Autodesk Inventor part; units mm, degrees
ref_plane "YZ Plane" through (0, 0, 0) normal (1, 0, 0) x (0, 1, 0)
ref_plane "XZ Plane" through (0, 0, 0) normal (0, 1, 0) x (-1, 0, 0)
ref_plane "XY Plane" through (0, 0, 0) normal (0, 0, 1) x (1, 0, 0)
sketch "Sketch1" plane through (0, 0, 0) normal (0, 1, 0) x (-1, 0, 0)
  line L0 (-12.7, -12.7) -> (12.7, -12.7)
  line L1 (12.7, -12.7) -> (12.7, 12.7)
  line L2 (12.7, 12.7) -> (-12.7, 12.7)
  line L3 (-12.7, 12.7) -> (-12.7, -12.7)
  line L4 (-12.7, -12.7) -> (12.7, 12.7) construction
  line L5 (12.7, -12.7) -> (-12.7, 12.7) construction
  line L6 (-10.9728, -10.9728) -> (10.9728, -10.9728)
  line L7 (10.9728, -10.9728) -> (10.9728, 10.9728)
  line L8 (10.9728, 10.9728) -> (-10.9728, 10.9728)
  line L9 (-10.9728, 10.9728) -> (-10.9728, -10.9728)
  line L10 (-10.9728, -10.9728) -> (10.9728, 10.9728) construction
  line L11 (10.9728, -10.9728) -> (-10.9728, 10.9728) construction
  point P0 (0, 0)
  dimension "d0" = 25.4
  dimension "d2" = 25.4
  dimension "d3" = 1.7272
  dimension "d4" = 1.7272
extrude "Extrusion1" add sketch "Sketch1" along normal blind 352.425
sketch "Sketch2" plane through (12.7, 0, 12.7) normal (1, 0, 0) x (0, 0, -1)
  line L0 (0, 352.425) -> (25.4, 352.425)
  line L1 (0, 0) -> (0, 352.425)
  point P0 (12.7, 0)
  point P1 (12.7, 339.725)
  dimension "d7" = 12.7
  dimension "d8" = 12.7
hole "Hole1" at (12.7, 339.725, 0) direction (-1, 0, 0) diameter 6.35 end through all
sketch "Sketch4" plane through (-12.7, 0, 12.7) normal (0, 0, 1) x (1, 0, 0)
  line L0 (0, 0) -> (25.4, 0)
  line L1 (25.4, 0) -> (25.4, 352.425)
  point P0 (12.7, 0)
  point P1 (12.7, 12.7)
  dimension "d25" = 12.7
  dimension "d26" = 12.7
hole "Hole3" at (0, 12.7, 12.7) direction (0, 0, -1) diameter 6.35 end through all
sketch "Sketch5" plane through (12.7, 0, -12.7) normal (0, 0, -1) x (-1, 0, 0)
  line L0 (0, 0) -> (25.4, 0)
  line L1 (25.4, 0) -> (25.4, 352.425)
  line L2 (0, 352.425) -> (25.4, 352.425)
  point P0 (12.7, 0)
  point P1 (12.7, 203.2)
  point P2 (12.7, 152.4)
  dimension "d34" = 50.8
  dimension "d36" = 152.4
  dimension "d38" = 149.225
  dimension "d39" = 352.425
  dimension "d40" = 12.7
  dimension "d41" = 12.7
hole "Hole4" at (0, 203.2, -12.7) at (0, 152.4, -12.7) direction (0, 0, 1) diameter 6.35 end through all
properties part number "BAseBAr" material "Aluminum 6061"
Geometry: final body of the model. Coordinates: model frame, mm. A direction names the side the tool comes from. Give positions to 0.01 mm unless a question says otherwise; leave off trailing zeros. Write each loop counter-clockwise with the first axis right and the second up, starting at its lowest first coordinate (ties: lowest second). Pieces come first, ordered by that corner, then holes. Notation, with made-up numbers: (44, -10.75) -> (61, -10.75) arc R10 cw to (61, 4.25) -> close; hole circle Ø11 at (-31, 26.5). An arc over 180 degrees is marked (long way). Answer as a JSON object with one key per item and string values.
1. Cut plane C-C on y = 12.7. Output: boundary loops of the cut face in (x, z) (3 decimals), and give its area (3 significant figures).
Ans:
{"outline": "(-12.7, -12.7) -> (-3.175, -12.7) -> (-3.175, -10.973) -> (-10.973, -10.973) -> (-10.973, 10.973) -> (-3.175, 10.973) -> (-3.175, 12.7) -> (-12.7, 12.7) -> close; (3.175, -12.7) -> (12.7, -12.7) -> (12.7, 12.7) -> (3.175, 12.7) -> (3.175, 10.973) -> (10.973, 10.973) -> (10.973, -10.973) -> (3.175, -10.973) -> close", "area": "142 mm^2"}
2. Ray query, probe 1 along Y at (x, z) = (0, 11.95) (3 decimals); probe 2 along X at (y, z) = (209, -3.25). Return the intervals inside material, ascending. Write a range as from..to.
Ans:
{"probe 1": "y = 0..9.525, 15.875..149.225, 155.575..200.025, 206.375..352.425", "probe 2": "x = -12.7..-10.97, 10.97..12.7"}
3. Contact query for a flat-ended pin moving along its axis: pin 1 (8.5 mm diameter, centred on y = 339.725, z = 0, fed in from -X). Output: stop coordinate, or through.
Ans:
{"pin 1": "stops at x = -12.7"}
4. Mould query, pull axis Z, two halves, no side actions, for faces 1 (the flat face through (0, 174, -10.973)), 2 (the cylindrical face through (1.22, 206.13, 11.85)), 3 (the flat face through (0, 174, 12.7)). Classes: pulls with the +Z half, pulls with the -Z half, needs draft (parallel to the pull), parting line crosses it, or undercut.
Ans:
{"face 1": "undercut", "face 2": "needs draft", "face 3": "pulls with the +Z half"}
5. Cut plane B-B on z = 6.75. Output: boundary loops of the cut face in (x, y) (3 decimals).
Ans:
{"outline": "(-12.7, 0) -> (-10.973, 0) -> (-10.973, 352.425) -> (-12.7, 352.425) -> close; (10.973, 0) -> (12.7, 0) -> (12.7, 352.425) -> (10.973, 352.425) -> close"}
6. Cut plane A-A on x = -7.5. Output: boundary loops of the cut face in (y, z) (3 decimals).
Ans:
{"outline": "(0, -12.7) -> (352.425, -12.7) -> (352.425, -10.973) -> (0, -10.973) -> close; (0, 10.973) -> (352.425, 10.973) -> (352.425, 12.7) -> (0, 12.7) -> close"}
7. Access query for faces 4 (the cylindrical face through (11.82, 337.05, -1.71)), 5 (the flat face through (0, 174, 10.973)). Directions: +Z, -Z, +X, -X, +Y, -Y. A direction counts if a zero-diameter tool reaches every point of the face in a straight line with its end or side. Return the directions, or none.
Ans:
{"face 4": "+X, -X", "face 5": "+Y, -Y"}
8. Cut plane D-D on y = 237. Output: boundary loops of the cut face in (x, z).
Ans:
{"outline": "(-12.7, -12.7) -> (12.7, -12.7) -> (12.7, 12.7) -> (-12.7, 12.7) -> close; hole (-10.97, -10.97) -> (10.97, -10.97) -> (10.97, 10.97) -> (-10.97, 10.97) -> close"}
